Model file for the job. Use its own axes, mm. Face numbers are marked on the shaded views. Round coordinates to 2 decimals unless told otherwise and drop trailing zeros. Write each loop counter-clockwise with the first axis right and the second up, starting at its lowest first coordinate (ties: lowest second). Pieces come first, ordered by that corner, then holes. Notation, with made-up numbers: (22, 12) - (63, 12) arc R21 cw to (63, 33) - close; hole circle Ø10 at (-37.75, 1). An arc over 180 degrees is marked (long way). Answer as a JSON object with one key per item and string values. Group by question number.
from build123d import *

# Parameters (mm, degrees)
SKETCH_1_W          = 52
SKETCH_1_H          = 52
SKETCH_1_R          = 15
SKETCH_1_R_2        = 1.6
EXTRUDE_1_DEPTH     = 80
SKETCH_2_R          = 1.6
SKETCH_2_R_2        = 15
CUT_EXTRUDE_1_DEPTH = 61


with BuildPart() as part:
    # 草图1 → 凸台-拉伸1 (new body)
    with BuildSketch(Plane.XY):
        with Locations((19.85443038, -6.661392405)):
            Rectangle(SKETCH_1_W, SKETCH_1_H)
        with Locations((19.85443038, -6.661392405)):
            Circle(SKETCH_1_R, mode=Mode.SUBTRACT)
        with Locations((35.35443038, 8.838607595)):
            Circle(SKETCH_1_R_2, mode=Mode.SUBTRACT)
        with Locations((35.35443038, -22.161392405)):
            Circle(SKETCH_1_R_2, mode=Mode.SUBTRACT)
        with Locations((4.35443038, -22.161392405)):
            Circle(SKETCH_1_R_2, mode=Mode.SUBTRACT)
        with Locations((4.35443038, 8.838607595)):
            Circle(SKETCH_1_R_2, mode=Mode.SUBTRACT)
    extrude(amount=EXTRUDE_1_DEPTH)

    # 草图2 → 切除-拉伸1 (cut)
    with BuildSketch(Plane.XY.offset(80)):
        Polygon((3.65443038, 14.538607595), (-1.34556962, 14.538607595), (-1.34556962, 9.538607595), (-6.14556962, 9.538607595), (-6.14556962, -22.861392405), (-1.34556962, -22.861392405), (-1.34556962, -27.861392405), (3.65443038, -27.861392405), (3.65443038, -32.661392405), (36.05443038, -32.661392405), (36.05443038, -27.861392405), (41.05443038, -27.861392405), (41.05443038, -22.861392405), (45.85443038, -22.861392405), (45.85443038, 9.538607595), (41.05443038, 9.538607595), (41.05443038, 14.538607595), (36.05443038, 14.538607595), (36.05443038, 19.338607595), (3.65443038, 19.338607595), align=None)
        with Locations((4.35443038, -22.161392405)):
            Circle(SKETCH_2_R, mode=Mode.SUBTRACT)
        with Locations((35.35443038, -22.161392405)):
            Circle(SKETCH_2_R, mode=Mode.SUBTRACT)
        with Locations((4.35443038, 8.838607595)):
            Circle(SKETCH_2_R, mode=Mode.SUBTRACT)
        with Locations((19.85443038, -6.661392405)):
            Circle(SKETCH_2_R_2, mode=Mode.SUBTRACT)
        with Locations((35.35443038, 8.838607595)):
            Circle(SKETCH_2_R, mode=Mode.SUBTRACT)
    extrude(amount=-CUT_EXTRUDE_1_DEPTH, mode=Mode.SUBTRACT)


solid = part.part
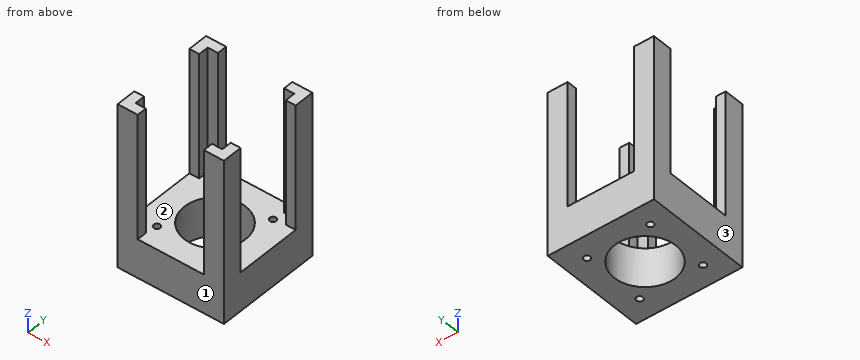
(1) Flat gauge pins, fed straight in: pin 1 (10 mm diameter, centred on x = 28, z = 58, fed in from +Y); pin 2 (12 mm diameter, centred on x = 29.5, y = 7.5, fed in from +Z). Where does each tip first touch, or does it go through?
(2) Slice it at D-D (y = 13). Write the cut outline in (x, z), then the cut area to 3 significant figures.
(3) Slice it at B-B (y = 1.5). Write the cut outline in (x, z).
(4) Drill centre lines: line 1 (Y direction, x = 41.5, z = 40.5); line 2 (X direction, y = -30.5, z = 67.5); line 3 (Y direction, x = 38, z = 44). Where is each one in solid material? Low to high. Write a range as from..to.
(5) Slice it at A-A (z = 20.5). Write the cut outline in (x, y), then the cut area to 3 significant figures.
(6) Pull direction Y, two halves, no side cores. Call the marked faces 1, 2 and 3: pulls with the +Y half, pulls with the -Y half, needs draft (parallel to the pull), parting line crosses it, or undercut.
(7) Slice it at C-C (x = 29.5). Write the cut outline in (y, z), then the cut area to 3 significant figures.
Answer:
{
 "1": {"pin 1": "through", "pin 2": "z = 19"},
 "2": {"outline": "(-6.15, 0) - (45.85, 0) - (45.85, 80) - (41.05, 80) - (41.05, 19) - (-1.35, 19) - (-1.35, 80) - (-6.15, 80) - close", "area": "1,570 mm²"},
 "3": {"outline": "(-6.15, 0) - (7.27, 0) - (7.27, 19) - (-6.15, 19) - close; (32.44, 0) - (45.85, 0) - (45.85, 19) - (32.44, 19) - close"},
 "4": {"line 1": "-32.66..-22.86, 9.54..19.34", "line 2": "-6.15..3.65, 36.05..45.85", "line 3": "-32.66..-27.86, 14.54..19.34"},
 "5": {"outline": "(-6.15, -32.66) - (3.65, -32.66) - (3.65, -27.86) - (-1.35, -27.86) - (-1.35, -22.86) - (-6.15, -22.86) - close; (-6.15, 9.54) - (-1.35, 9.54) - (-1.35, 14.54) - (3.65, 14.54) - (3.65, 19.34) - (-6.15, 19.34) - close; (36.05, -32.66) - (45.85, -32.66) - (45.85, -22.86) - (41.05, -22.86) - (41.05, -27.86) - (36.05, -27.86) - close; (36.05, 14.54) - (41.05, 14.54) - (41.05, 9.54) - (45.85, 9.54) - (45.85, 19.34) - (36.05, 19.34) - close", "area": "284 mm²"},
 "6": {"face 1": "pulls with the -Y half", "face 2": "undercut", "face 3": "needs draft"},
 "7": {"outline": "(-32.66, 0) - (-18.15, 0) - (-18.15, 19) - (-32.66, 19) - close; (4.83, 0) - (19.34, 0) - (19.34, 19) - (4.83, 19) - close", "area": "551 mm²"}
}
